Autodesk Inventor part; units mm, degrees
ref_plane "1_XY" through (0, 0, 0) normal (1, 0, 0) x (0, 0, -1)
ref_plane "1_YZ" through (0, 0, 0) normal (0, 0, -1) x (0, 1, 0)
ref_plane "1_ZX" through (0, 0, 0) normal (0, 1, 0) x (1, 0, 0)
sketch "Sketch_5" plane through (0, 0, 0) normal (1, 0, 0) x (0, 1, 0)
  arc A0 (-3.0551, -2.7867) -> (-3.0551, 2.7867) centre (0.35, 0) ccw
  arc A1 (-4.2933, 2.2) -> (-3.0551, 2.7867) centre (-4.2933, 3.8) ccw
  line L0 (-4.2933, 2.2) -> (-4.75, 2.2)
  arc A2 (-4.75, 2.2) -> (-6.35, 0.6) centre (-4.75, 0.6) ccw
  line L1 (-6.35, 0.6) -> (-6.35, 0.025)
  line L2 (-6.35, 0.025) -> (-5.25, 0.025)
  line L3 (-5.25, 0.025) -> (-5.25, 0.9)
  arc A3 (-4.25, 0.9) -> (-5.25, 0.9) centre (-4.75, 0.9) ccw
  line L4 (-4.25, 0.9) -> (-4.25, 0.025)
  line L5 (-4.25, 0.025) -> (-3.3499, 0.025)
  arc A4 (-3.3499, -0.025) -> (-3.3499, 0.025) centre (0, 0) ccw
  line L6 (-3.3499, -0.025) -> (-4.25, -0.025)
  line L7 (-4.25, -0.025) -> (-4.25, -0.9)
  arc A5 (-5.25, -0.9) -> (-4.25, -0.9) centre (-4.75, -0.9) ccw
  line L8 (-5.25, -0.9) -> (-5.25, -0.025)
  line L9 (-5.25, -0.025) -> (-6.35, -0.025)
  line L10 (-6.35, -0.025) -> (-6.35, -0.6)
  arc A6 (-6.35, -0.6) -> (-4.75, -2.2) centre (-4.75, -0.6) ccw
  line L11 (-4.75, -2.2) -> (-4.2933, -2.2)
  arc A7 (-3.0551, -2.7867) -> (-4.2933, -2.2) centre (-4.2933, -3.8) ccw
extrude "Extrusion1" add sketch "Sketch_5" along normal mid plane 0.8
ref_plane "1_XY" through (0, 0, 0) normal (1, 0, 0) x (0, 0, -1)
ref_plane "1_YZ" through (0, 0, 0) normal (0, 0, -1) x (0, 1, 0)
ref_plane "1_ZX" through (0, 0, 0) normal (0, 1, 0) x (1, 0, 0)
ref_plane "combination_module_XY" through (0.4, 0, 0) normal (1, 0, 0) x (0, 0, -1)
ref_plane "combination_module_YZ" through (0.4, 0, 0) normal (0, 0, -1) x (0, 1, 0)
ref_plane "combination_module_ZX" through (0.4, 0, 0) normal (0, 1, 0) x (1, 0, 0)
properties part number "STWN7" material "Steel"
Could you check a few things on this model? Use its own coordinates, in mm. Give positions to 0.01 mm unless a question says otherwise; leave off trailing zeros. Order: outer loops, then holes, each group sorted by start corner. A loop starts at its lowest first (then second) coordinate and runs counter-clockwise, first axis right, second up.
Item 1: I'm going to push flat-ended pins straight in: pin 1 (4 mm diameter, centred on y = 0, z = -3, fed in from +X); pin 2 (2 mm diameter, centred on y = -1, z = 2, fed in from +X) (3 decimals). Where does each tip first touch, or does it pass through?
Item 2: If we section it at D-D, the plane y = 3.75: Write out the boundary of the cut face in (x, z), plus the area to 3 significant figures.
Item 3: If we section it at C-C, the plane y = 0.35: Write out the boundary of the cut face in (x, z), plus the area to 3 significant figures.
Item 4: If we section it at A-A, the plane z = -2.5: Write out the boundary of the cut face in (x, y), plus the area to 3 significant figures.
Item 5: If we section it at B-B, the plane x = -0.1: Write out the boundary of the cut face in (y, z) (3 decimals), plus the area to 3 significant figures.
Item 6: If we mould it in two halves opening along Z, with no side actions, what happens to faces 1 (the face through (-0.01, -5.87, -1.74)), 2 (the face through (-0.006, 3.347, 0.147)), 3 (the face through (-0.01, -5.89, 1.72)), 4 (the face through (-0.4, -3, 2))? For each: pulls with the +Z half, pulls with the -Z half, needs draft (parallel to the pull), parting line crosses it, or undercut.
Item 7: I need wall thicknesses on line 1 (Y direction, x = 0.35, z = -1); line 2 (Y direction, x = 0.35, z = -0.75); line 3 (Z direction, x = 0.1, y = 0). Which ranges of each line are inside material? Lowest first, please.
Values:
1. pin 1: stops at x = 0.4
1. pin 2: passes through
2. outline: (-0.4, -2.79) - (0.4, -2.79) - (0.4, 2.79) - (-0.4, 2.79) - close
2. area: 4.47 mm2
3. outline: (-0.4, -4.4) - (0.4, -4.4) - (0.4, -3.33) - (-0.4, -3.33) - close; (-0.4, 3.33) - (0.4, 3.33) - (0.4, 4.4) - (-0.4, 4.4) - close
3. area: 1.71 mm2
4. outline: (-0.4, -3.36) - (0.4, -3.36) - (0.4, -2.23) - (-0.4, -2.23) - close; (-0.4, 2.23) - (0.4, 2.23) - (0.4, 3.97) - (-0.4, 3.97) - close
4. area: 2.30 mm2
5. outline: (-6.35, -0.6) arc R1.6 ccw to (-4.75, -2.2) - (-4.293, -2.2) arc R1.6 cw to (-3.055, -2.787) arc R4.4 ccw (long way) to (-3.055, 2.787) arc R1.6 cw to (-4.293, 2.2) - (-4.75, 2.2) arc R1.6 ccw to (-6.35, 0.6) - (-6.35, 0.025) - (-5.25, 0.025) - (-5.25, 0.9) arc R0.5 cw to (-4.25, 0.9) - (-4.25, 0.025) - (-3.35, 0.025) arc R3.35 cw (long way) to (-3.35, -0.025) - (-4.25, -0.025) - (-4.25, -0.9) arc R0.5 cw to (-5.25, -0.9) - (-5.25, -0.025) - (-6.35, -0.025) - close
5. area: 32.9 mm2
6. face 1: pulls with the -Z half
6. face 2: undercut
6. face 3: pulls with the +Z half
6. face 4: needs draft
7. line 1: y = -6.3 to -5.24, -4.26 to -3.2, 3.2 to 4.63
7. line 2: y = -6.34 to -5.25, -4.25 to -3.26, 3.26 to 4.69
7. line 3: z = -4.39 to -3.35, 3.35 to 4.39
